For this review, use the dimensioned drawing (mm, ordinates from the lowest corner) and the shaded views. A direction names the side the tool comes from. Round coordinates to 2 decimals unless told otherwise and drop trailing zeros. Write each loop counter-clockwise with the first axis right and the second up, starting at its lowest first coordinate (ties: lowest second). Pieces come first, ordered by that corner, then holes. Notation, with made-up numbers: M 83.25,8.5 L 130.25,8.5 A16 cw 130.25,25.5 Z; hole C -1,78 d11. An arc over 180 degrees is marked long. One line per question, with ' | ' between items.
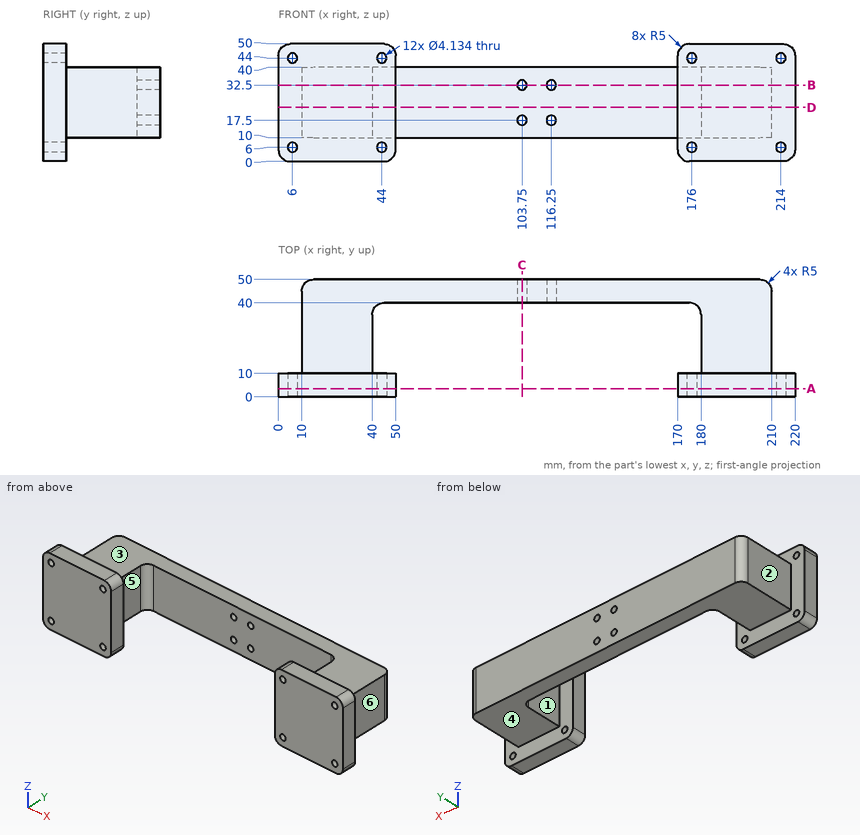
Item 1: To check wall thickness, follow line 1 along Z through (x, y) = (6, 4); line 2 along Z through (x, y) = (116.25, 43.5); line 3 along X through (y, z) = (4, 18). State the ranges of each line that lie inside material, in increasing order. Write a range as from..to.
Results:
line 1: 0..3.93, 8.07..41.93, 46.07..50 | line 2: 10..15.43, 19.57..30.43, 34.57..40 | line 3: 0..50, 170..220
Item 2: Take a section at B-B (z = 32.5). Write out the cut boundary in (x, y), then the cut area to 3 significant figures.
Results:
outline: M 0,0 L 50,0 L 50,10 L 40,10 L 40,35 A5 cw 45,40 L 101.68,40 L 101.68,50 L 15,50 A5 ccw 10,45 L 10,10 L 0,10 Z; M 105.82,40 L 114.18,40 L 114.18,50 L 105.82,50 Z; M 118.32,40 L 175,40 A5 cw 180,35 L 180,10 L 170,10 L 170,0 L 220,0 L 220,10 L 210,10 L 210,45 A5 ccw 205,50 L 118.32,50 Z | area: 4,720 mm2
Item 3: Take a section at A-A (y = 3.5). State how many separate pieces and enclosed holes the cut face has, then the cut area to 3 significant figures.
Results:
separate pieces: 2 | enclosed holes: 8 | area: 4,850 mm2
Item 4: Mouldability with a two-part tool opening along X and no side actions: class the marked faces 1, 2 and 3 as +X half, -X half, draft (parallel to the pull), parting line (faces both ways), or undercut.
Results:
face 1: undercut | face 2: -X half | face 3: draft
Item 5: Insertion check: pin 1 Ø3.5 at (x, z) = (103.75, 32.5) entering from -Y; pin 2 Ø6.5 at (x, z) = (176, 6) entering from -Y; pin 3 Ø8 at (x, y) = (40.5, 23.5) entering from +Z; pin 4 Ø8 at (y, z) = (34.5, 27) entering from -X. Each pin has a flat end and moves straight along its axis. Give the tip position at first contact, or say it passes through.
Results:
pin 1: through | pin 2: y = 0 | pin 3: z = 40 | pin 4: x = 10
Item 6: Machinability: for the marked faces 4, 5 and 6, which of the approach directions +Z, -Z, +X, -X, +Y, -Y give a long, thin tool a straight path to every point of the face, cutting with its end or side? Answer none if there is none.
Results:
face 4: -Z, +X, -X, +Y | face 5: +Z, -Z | face 6: +Z, -Z, +X, +Y
Item 7: Take a section at C-C (x = 103.75). Write out the cut boundary in (y, z).
Results:
outline: M 40,10 L 50,10 L 50,15.43 L 40,15.43 Z; M 40,19.57 L 50,19.57 L 50,30.43 L 40,30.43 Z; M 40,34.57 L 50,34.57 L 50,40 L 40,40 Z
Item 8: Take a section at D-D (z = 23). Write out the cut boundary in (x, y).
Results:
outline: M 0,0 L 50,0 L 50,10 L 40,10 L 40,35 A5 cw 45,40 L 175,40 A5 cw 180,35 L 180,10 L 170,10 L 170,0 L 220,0 L 220,10 L 210,10 L 210,45 A5 ccw 205,50 L 15,50 A5 ccw 10,45 L 10,10 L 0,10 Z
